from build123d import *

# Parameters (mm, degrees)
SKETCH1_R                = 2.5
BOSS_EXTRUDE1_DEPTH      = 16
SKETCH2_R                = 1.5875
BOSS_EXTRUDE2_DEPTH      = 16
BOSS_EXTRUDE2_DEPTH_BACK = 20


with BuildPart() as part:
    # Sketch1 → Boss-Extrude1 (new body)
    with BuildSketch(Plane.XY):
        Circle(SKETCH1_R)
    extrude(amount=BOSS_EXTRUDE1_DEPTH)

    # Sketch2 → Boss-Extrude2 (add, two sides)
    with BuildSketch(Plane.XY.offset(16)) as boss_extrude2_sk:
        Circle(SKETCH2_R)
    extrude(amount=BOSS_EXTRUDE2_DEPTH)
    extrude(boss_extrude2_sk.sketch, amount=-BOSS_EXTRUDE2_DEPTH_BACK)


solid = part.part
CAD build for the part. Positions are in the model's coordinates, mm. A direction names the side the tool comes from. Give positions to 0.01 mm unless a question says otherwise; leave off trailing zeros. Order: outer loops, then holes, each group sorted by start corner. A loop starts at its lowest first (then second) coordinate and runs counter-clockwise, first axis right, second up. Notation, with made-up numbers: (8.5, 55.25) - (62.5, 55.25) arc R8 cw to (62.5, 62.25) - close; hole circle Ø11 at (72.5, -6.75). An arc over 180 degrees is marked (long way). Answer in a Markdown table with one row per item.
1. Probe probe 1 along X at (y, z) = (-0.15, -1); probe 2 along Z at (x, y) = (-0.7, 2.3); probe 3 along X at (y, z) = (1, 26.5). List the from-to ranges inside material, lowest first. Write a range as [from, to].
Data:
| item | result |
|---|---|
| probe 1 | x = [-1.58, 1.58] |
| probe 2 | z = [0, 16] |
| probe 3 | x = [-1.23, 1.23] |
2. Tool access for faces 1 (the flat face through (0, 0, 32)), 2 (the cylindrical face through (-0.34, -1.55, -1.97)), 3 (the cylindrical face through (-0.34, -1.55, 23.89)): list every direction of +Z, -Z, +X, -X, +Y, -Y with a clear straight run to the whole face (end or side of a thin tool).
Data:
| item | result |
|---|---|
| face 1 | +Z, +X, -X, +Y, -Y |
| face 2 | -Z |
| face 3 | +Z |
3. Saw through at C-C, the plane z = 29. Give the cut face in (x, y) (1 decimal).
Data:
| item | result |
|---|---|
| outline | circle Ø3.2 at (0, 0) |
4. Saw through at D-D, the plane z = 13. Give the cut face in (x, y), plus the area to 3 significant figures.
Data:
| item | result |
|---|---|
| outline | circle Ø5 at (0, 0) |
| area | 19.6 mm² |
5. Saw through at A-A, the plane y = 0. Give the cut face in (x, z), plus the area to 4 significant figures.
Data:
| item | result |
|---|---|
| outline | (-2.5, 0) - (-1.59, 0) - (-1.59, -4) - (1.59, -4) - (1.59, 0) - (2.5, 0) - (2.5, 16) - (1.59, 16) - (1.59, 32) - (-1.59, 32) - (-1.59, 16) - (-2.5, 16) - close |
| area | 143.5 mm² |
6. Flat gauge pins, fed straight in: pin 1 (2 mm diameter, centred on x = -1, z = 21, fed in from +Y); pin 2 (1 mm diameter, centred on x = -1.5, z = 22, fed in from +Y); pin 3 (1 mm diameter, centred on x = 1.5, z = 11.5, fed in from -Y). Where does each tip first touch, or does it go through?
Data:
| item | result |
|---|---|
| pin 1 | stops at y = 1.59 |
| pin 2 | stops at y = 1.23 |
| pin 3 | stops at y = -2.29 |
